Could you check a few things on this drawing? It's one solid part, dimensions in mm from its lowest x, y, z. A direction names the side the tool comes from. Give positions to 0.01 mm unless a question says otherwise; leave off trailing zeros. Order: outer loops, then holes, each group sorted by start corner. A loop starts at its lowest first (then second) coordinate and runs counter-clockwise, first axis right, second up.
Item 1: Which directions (+Z, -Z, +X, -X, +Y, -Y) give clear straight access to the entire face, cutting with the end or side of a thin tool? Please do the marked faces 5 and 6.
Item 2: I want a section at A-A, the plane x = 57.15. Write out the boundary of the cut face in (y, z).
Item 3: If we mould it in two halves opening along X, with no side actions, what happens to the marked faces 1, 2, 3 and 4? For each: +X half, -X half, draft (parallel to the pull), parting line (faces both ways), or undercut.
Item 4: If I drill on line 1 along Z through (x, y) = (57.15, 1.75); line 2 along X through (y, z) = (47.5, 58.5), over which ranges is the centre line in solid material (lowest first)?
Item 5: I'm going to push a flat-ended pin straight in: pin 1 Ø3 at (x, y) = (18.5, 79.5) entering from +Z. Where does the tip first touch, or does it pass through?
Item 6: I want a section at C-C, the plane y = 13. Write out the boundary of the cut face in (x, z), then the cut area to 3 significant figures.
Item 7: I want a section at B-B, the plane z = 33. Write out the boundary of the cut face in (x, y), then the cut area to 3 significant figures.
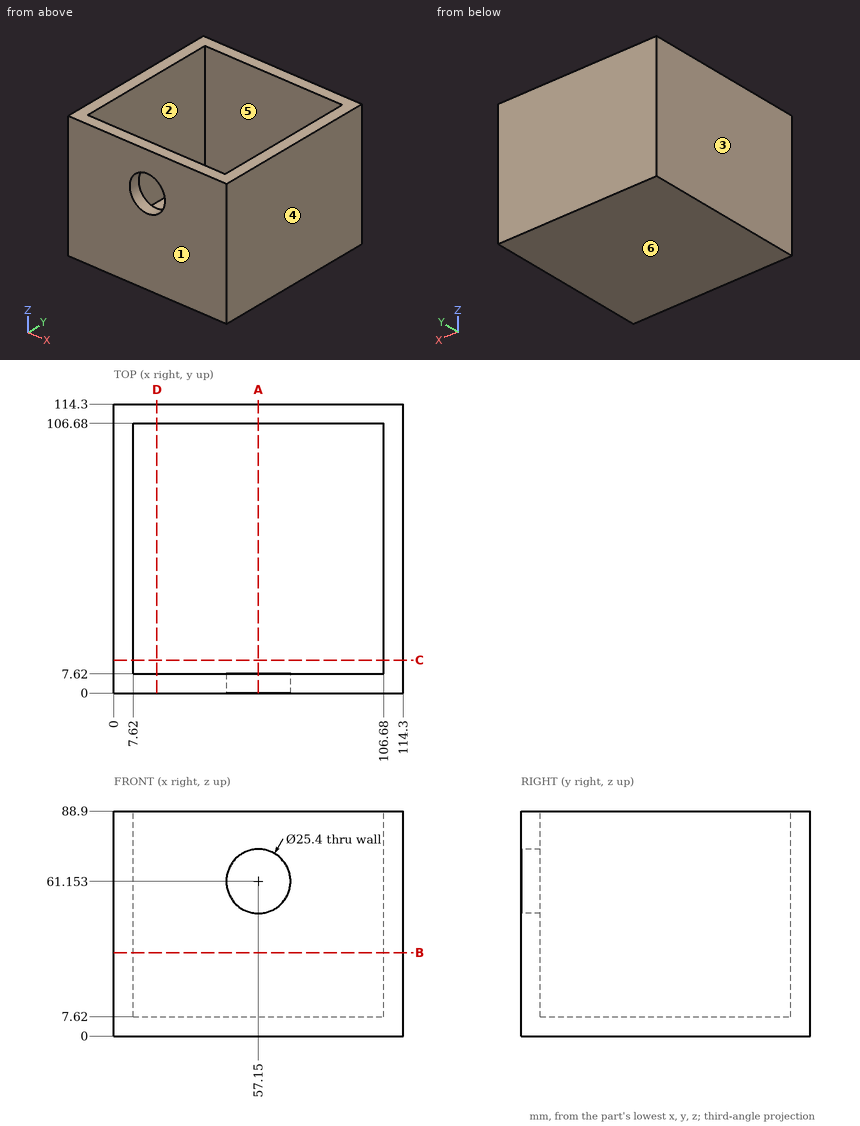
Results list:
1. face 5: +Z
1. face 6: -Z, +X, -X, +Y, -Y
2. outline: (0, 0) - (114.3, 0) - (114.3, 88.9) - (106.68, 88.9) - (106.68, 7.62) - (7.62, 7.62) - (7.62, 48.45) - (0, 48.45) - close; (0, 73.85) - (7.62, 73.85) - (7.62, 88.9) - (0, 88.9) - close
3. face 1: draft
3. face 2: undercut
3. face 3: -X half
3. face 4: +X half
4. line 1: z = 0 to 48.45, 73.85 to 88.9
4. line 2: x = 0 to 7.62, 106.68 to 114.3
5. pin 1: stops at z = 7.62
6. outline: (0, 0) - (114.3, 0) - (114.3, 88.9) - (106.68, 88.9) - (106.68, 7.62) - (7.62, 7.62) - (7.62, 88.9) - (0, 88.9) - close
6. area: 2,110 mm2
7. outline: (0, 0) - (114.3, 0) - (114.3, 114.3) - (0, 114.3) - close; hole (7.62, 7.62) - (106.68, 7.62) - (106.68, 106.68) - (7.62, 106.68) - close
7. area: 3,250 mm2
